```python
from build123d import *

# Parameters (mm, degrees)
SKETCH1_W           = 2.8
SKETCH1_H           = 178.3
BOSS_EXTRUDE1_DEPTH = 11.8
CUT_EXTRUDE1_REACH  = 180.812
SKETCH2_R           = 2
LPATTERN1_COUNT     = 3
LPATTERN1_PITCH     = 82.5


with BuildPart() as part:
    # Sketch1 → Boss-Extrude1 (new body)
    with BuildSketch(Plane(origin=(0, 0, 0), x_dir=(0, 1, 0), z_dir=(0, 0, 1))):
        with Locations((1.5, 89.25)):
            Rectangle(SKETCH1_W, SKETCH1_H)
    extrude(amount=BOSS_EXTRUDE1_DEPTH)

    # Sketch2 → Cut-Extrude1 (cut, up to next)
    with BuildSketch(Plane(origin=(0, 2.9, 0), x_dir=(-1, 0, 0), z_dir=(0, 1, 0)), mode=Mode.PRIVATE) as cut_extrude1_sk1:
        with Locations(Location((171.75, 2.9, 0), (0, 0, 90))):
            Circle(SKETCH2_R)
    cut_extrude1_tool1 = extrude(cut_extrude1_sk1.sketch, amount=-CUT_EXTRUDE1_REACH, mode=Mode.PRIVATE) & part.part
    cut_extrude1 = cut_extrude1_tool1.solids().sort_by_distance((-171.75, 2.9, 2.9))[0]
    add(cut_extrude1, mode=Mode.SUBTRACT)

    # LPattern1: Cut-Extrude1 ×3
    with Locations(*[(i * LPATTERN1_PITCH, 0, 0) for i in range(1, LPATTERN1_COUNT)]):
        add(cut_extrude1, mode=Mode.SUBTRACT)


solid = part.part
```
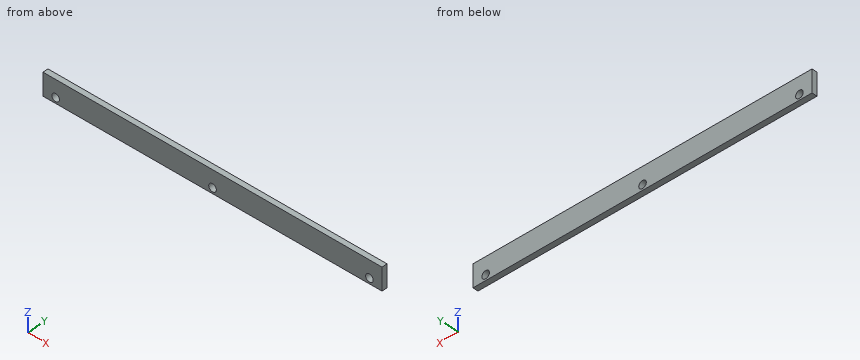
Here's how the part is built. I have some questions about the finished solid (model axes, mm). Round coordinates to 2 decimals unless told otherwise and drop trailing zeros. Loops run counter-clockwise (first coordinate to the right, second up) from the corner with the lowest first, then second, coordinate; pieces in that order, holes last. Notation, with made-up numbers: (13.25, 89) -> (19.25, 89) arc R21 ccw to (19.25, 112) -> close; hole circle Ø4 at (-34, 82.5). An arc over 180 degrees is marked (long way). Answer as CSV lines item,"result". Start each with the question number.
1. I'm going to push a flat-ended pin straight in: P1, Ø1, axis at x = -31.5, y = 2.5, coming from the -Z side. Where does the tip first touch, or does it pass through?
2. Imagine slicing it at A-A on x = -89.25. Write out the boundary of the cut face in (y, z).
3. I need wall thicknesses on probe 1 along X at (y, z) = (1.2, 2.9); probe 2 along Z at (x, y) = (-6.75, 0.9); probe 3 along X at (y, z) = (1.4, 2). Which ranges of each line are inside material? Lowest first, please. Write a range as from..to.
4. Imagine slicing it at C-C on y = 2.25. Write out the boundary of the cut face in (x, z), plus the area to 3 significant figures.
5. Imagine slicing it at B-B on z = 2.9. Write out the boundary of the cut face in (x, y).
Solution:
1,P1,"z = 0"
2,outline,"(0.1, 0) -> (2.9, 0) -> (2.9, 0.9) -> (0.1, 0.9) -> close; (0.1, 4.9) -> (2.9, 4.9) -> (2.9, 11.8) -> (0.1, 11.8) -> close"
3,probe 1,"-178.4..-173.75, -169.75..-91.25, -87.25..-8.75, -4.75..-0.1"
3,probe 2,"0..0.9, 4.9..11.8"
3,probe 3,"-178.4..-173.54, -169.96..-91.04, -87.46..-8.54, -4.96..-0.1"
4,outline,"(-178.4, 0) -> (-0.1, 0) -> (-0.1, 11.8) -> (-178.4, 11.8) -> close; hole circle Ø4 at (-171.75, 2.9); hole circle Ø4 at (-89.25, 2.9); hole circle Ø4 at (-6.75, 2.9)"
4,area,"2,070 mm²"
5,outline,"(-178.4, 0.1) -> (-173.75, 0.1) -> (-173.75, 2.9) -> (-178.4, 2.9) -> close; (-169.75, 0.1) -> (-91.25, 0.1) -> (-91.25, 2.9) -> (-169.75, 2.9) -> close; (-87.25, 0.1) -> (-8.75, 0.1) -> (-8.75, 2.9) -> (-87.25, 2.9) -> close; (-4.75, 0.1) -> (-0.1, 0.1) -> (-0.1, 2.9) -> (-4.75, 2.9) -> close"
